Design review of the part built by this model. Coordinates are the model's own, in mm. Face numbers are marked on the shaded views. A direction names the side the tool comes from. Coordinates: 2 decimals unless noted, no trailing zeros. Write each loop counter-clockwise with the first axis right and the second up, starting at its lowest first coordinate (ties: lowest second). Pieces come first, ordered by that corner, then holes.
Q1. Take a section at C-C (y = -28.5). Give the boundary of the cut face in (x, z).
Q2. Insertion check: pin 1 (10 mm diameter, centred on y = -48.5, z = -11, fed in from +X); pin 2 (10 mm diameter, centred on y = -46.5, z = -28.5, fed in from -X); pin 3 (10 mm diameter, centred on y = -43.5, z = -17, fed in from -X). Each pin has a flat end and moves straight along its axis. Give the tip position at first contact, or say it passes through.
Q3. Take a section at B-B (z = 0). Give the boundary of the cut face in (x, y), and give its area (3 significant figures).
Q4. Take a section at A-A (x = 0). Give the boundary of the cut face in (y, z), and give its area (3 significant figures).
Q5. Machinability: for the marked faces 1 and 2, which of the approach directions +Z, -Z, +X, -X, +Y, -Y give a long, thin tool a straight path to every point of the face, cutting with its end or side? Answer none if there is none.
Q6. For probe 1 along Z at (x, y) = (0, -0.7); probe 2 along Z at (x, y) = (0, -47); probe 3 along Y at (x, z) = (39.5, 15.5), list the stretches that pass through material, from the lowest coordinate up.
Q7. Take a section at D-D (x = 23). Give the boundary of the cut face in (y, z), and give its area (3 significant figures).
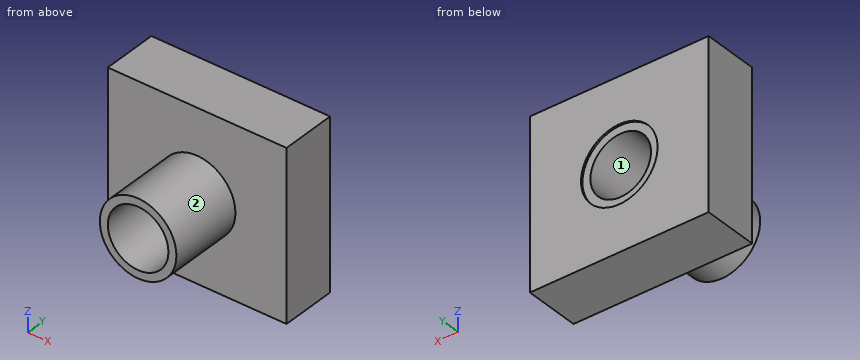
```python
from build123d import *

# Parameters (mm, degrees)
F0_W      = 99.465304
F0_H      = 93.672826
F1_DEPTH  = 30.734
F2_R      = 21.313315
F2_R_2    = 16.867253
F3_DEPTH  = 72.39
F4_DEPTH  = 1.016
F4_FACE_R = 16.867253
F6_DEPTH  = 76.708


with BuildPart() as f1:
    # F0 (on Front) → F1 (new body)
    with BuildSketch(Plane.XZ):
        Rectangle(F0_W, F0_H)
    extrude(amount=F1_DEPTH)

    # F2 (on Front) → F3 (join)
    with BuildSketch(Plane.XZ):
        Circle(F2_R)
        Circle(F2_R_2, mode=Mode.SUBTRACT)
    extrude(amount=F3_DEPTH)

    # F2 (on Front) → F4 (cut)
    with BuildSketch(Plane.XZ):
        Circle(F2_R)
        Circle(F2_R_2, mode=Mode.SUBTRACT)
    extrude(amount=F4_DEPTH, mode=Mode.SUBTRACT)

    # F4_face (on face) → F6 (cut)
    with BuildSketch(Plane(origin=(0, 0, 0), x_dir=(1, 0, 0), z_dir=(0, 1, 0))):
        Circle(F4_FACE_R)
    extrude(amount=-F6_DEPTH, mode=Mode.SUBTRACT)


solid = f1.part
```
Response:
1. outline: (-49.73, -46.84) - (49.73, -46.84) - (49.73, 46.84) - (-49.73, 46.84) - close; hole circle Ø33.73 at (0, 0)
2. pin 1: stops at x = 20.45
2. pin 2: passes through
2. pin 3: stops at x = -17.61
3. outline: (-49.73, -30.73) - (-21.31, -30.73) - (-21.31, -72.39) - (-16.87, -72.39) - (-16.87, -1.02) - (-21.31, -1.02) - (-21.31, 0) - (-49.73, 0) - close; (16.87, -72.39) - (21.31, -72.39) - (21.31, -30.73) - (49.73, -30.73) - (49.73, 0) - (21.31, 0) - (21.31, -1.02) - (16.87, -1.02) - close
3. area: 2,380 mm2
4. outline: (-72.39, -21.31) - (-30.73, -21.31) - (-30.73, -46.84) - (0, -46.84) - (0, -21.31) - (-1.02, -21.31) - (-1.02, -16.87) - (-72.39, -16.87) - close; (-72.39, 16.87) - (-1.02, 16.87) - (-1.02, 21.31) - (0, 21.31) - (0, 46.84) - (-30.73, 46.84) - (-30.73, 21.31) - (-72.39, 21.31) - close
4. area: 2,200 mm2
5. face 1: +Y, -Y
5. face 2: -Y
6. probe 1: z = -46.84 to -21.31, 21.31 to 46.84
6. probe 2: z = -21.31 to -16.87, 16.87 to 21.31
6. probe 3: y = -30.73 to 0
7. outline: (-30.73, -46.84) - (0, -46.84) - (0, 46.84) - (-30.73, 46.84) - close
7. area: 2,880 mm2
